For this review, take the finished solid that the model builds, in its own axes (mm). A direction names the side the tool comes from. Round coordinates to 2 decimals unless told otherwise and drop trailing zeros. Write each loop counter-clockwise with the first axis right and the second up, starting at its lowest first coordinate (ties: lowest second). Pieces come first, ordered by that corner, then holes. Notation, with made-up numbers: (39, 47.5) -> (50, 47.5) arc R19 ccw to (50, 60.5) -> close; hole circle Ø1 at (32.5, 40). An arc over 180 degrees is marked (long way). Answer in a Markdown table with one row per item.
from build123d import *

# Parameters (mm, degrees)
F1_DEPTH = 12.7
F3_DEPTH = 1.27
F4_DEPTH = 1.27
F5_W     = 15.24
F5_H     = 2.54
F6_DEPTH = 19.05


with BuildPart() as f1:
    # F0 (on Front) → F1 (new body, symmetric)
    with BuildSketch(Plane.XZ):
        Polygon((-22.86, 14.2980794165), (-31.115, 0), (0, 0), (0, 14.2980794165), align=None)
        Polygon((0, 14.2980794165), (0, 0), (31.115, 0), (22.86, 14.2980794165), align=None)
        Polygon((0, 0), (0, -14.2980794165), (39.37, -14.2980794165), (31.115, 0), align=None)
        Polygon((-31.115, 0), (-39.37, -14.2980794165), (0, -14.2980794165), (0, 0), align=None)
    extrude(amount=F1_DEPTH, both=True)

    # F2 (on face) → F3 (cut)
    with BuildSketch(Plane.XZ.offset(12.7)):
        with BuildLine():
            Line((0, -11.0009658396), (-0.00127, -10.9987661351))
            ThreePointArc((-0.00127, -10.9987661351), (-0.0021997045, -10.9996958396), (-0.00254, -11.0009658396))
            Line((-0.00254, -11.0009658396), (0, -11.0009658396))
        make_face()
        with BuildLine():
            ThreePointArc((-6.34873, -0.0046429161), (-6.35, -0.0049832116), (-6.35127, -0.0046429161))
            Line((-6.35127, -0.0046429161), (-12.7, -11.0009658396))
            Line((-12.7, -11.0009658396), (-0.00254, -11.0009658396))
            ThreePointArc((-0.00254, -11.0009658396), (-0.0021997045, -10.9996958396), (-0.00127, -10.9987661351))
            Line((-0.00127, -10.9987661351), (-6.34873, -0.0046429161))
        make_face()
        with BuildLine():
            Line((-6.34873, -0.0046429161), (-6.35, -0.0024432116))
            Line((-6.35, -0.0024432116), (-6.35127, -0.0046429161))
            ThreePointArc((-6.35127, -0.0046429161), (-6.35, -0.0049832116), (-6.34873, -0.0046429161))
        make_face()
    extrude(amount=-F3_DEPTH, mode=Mode.SUBTRACT)

    # F2 (on face) → F4 (cut)
    with BuildSketch(Plane.XZ.offset(12.7)):
        with BuildLine():
            Line((6.34873, -0.0002435071), (0, 10.9960794165))
            Line((0, 10.9960794165), (-6.34873, -0.0002435071))
            ThreePointArc((-6.34873, -0.0002435071), (-6.3478002955, -0.0011732116), (-6.34746, -0.0024432116))
            Line((-6.34746, -0.0024432116), (6.34746, -0.0024432116))
            ThreePointArc((6.34746, -0.0024432116), (6.3478002955, -0.0011732116), (6.34873, -0.0002435071))
        make_face()
        with BuildLine():
            ThreePointArc((-6.34873, -0.0046429161), (-6.35, -0.0049832116), (-6.35127, -0.0046429161))
            Line((-6.35127, -0.0046429161), (-12.7, -11.0009658396))
            Line((-12.7, -11.0009658396), (-0.00254, -11.0009658396))
            ThreePointArc((-0.00254, -11.0009658396), (-0.0021997045, -10.9996958396), (-0.00127, -10.9987661351))
            Line((-0.00127, -10.9987661351), (-6.34873, -0.0046429161))
        make_face()
        with BuildLine():
            Line((12.7, -11.0009658396), (6.35127, -0.0046429161))
            ThreePointArc((6.35127, -0.0046429161), (6.35, -0.0049832116), (6.34873, -0.0046429161))
            Line((6.34873, -0.0046429161), (0.00127, -10.9987661351))
            ThreePointArc((0.00127, -10.9987661351), (0.0021997045, -10.9996958396), (0.00254, -11.0009658396))
            Line((0.00254, -11.0009658396), (12.7, -11.0009658396))
        make_face()
        with BuildLine():
            Line((-6.34873, -0.0046429161), (-6.35, -0.0024432116))
            Line((-6.35, -0.0024432116), (-6.35127, -0.0046429161))
            ThreePointArc((-6.35127, -0.0046429161), (-6.35, -0.0049832116), (-6.34873, -0.0046429161))
        make_face()
        with BuildLine():
            Line((-6.34746, -0.0024432116), (-6.35, -0.0024432116))
            Line((-6.35, -0.0024432116), (-6.34873, -0.0046429161))
            ThreePointArc((-6.34873, -0.0046429161), (-6.3478002955, -0.0037132116), (-6.34746, -0.0024432116))
        make_face()
        with BuildLine():
            ThreePointArc((-6.34746, -0.0024432116), (-6.3478002955, -0.0011732116), (-6.34873, -0.0002435071))
            Line((-6.34873, -0.0002435071), (-6.35, -0.0024432116))
            Line((-6.35, -0.0024432116), (-6.34746, -0.0024432116))
        make_face()
        with BuildLine():
            Line((6.35, -0.0024432116), (6.34873, -0.0002435071))
            ThreePointArc((6.34873, -0.0002435071), (6.3478002955, -0.0011732116), (6.34746, -0.0024432116))
            Line((6.34746, -0.0024432116), (6.35, -0.0024432116))
        make_face()
        with BuildLine():
            Line((6.34873, -0.0046429161), (6.35, -0.0024432116))
            Line((6.35, -0.0024432116), (6.34746, -0.0024432116))
            ThreePointArc((6.34746, -0.0024432116), (6.3478002955, -0.0037132116), (6.34873, -0.0046429161))
        make_face()
        with BuildLine():
            Line((6.35127, -0.0046429161), (6.35, -0.0024432116))
            Line((6.35, -0.0024432116), (6.34873, -0.0046429161))
            ThreePointArc((6.34873, -0.0046429161), (6.35, -0.0049832116), (6.35127, -0.0046429161))
        make_face()
        with BuildLine():
            Line((0, -11.0009658396), (-0.00127, -10.9987661351))
            ThreePointArc((-0.00127, -10.9987661351), (-0.0021997045, -10.9996958396), (-0.00254, -11.0009658396))
            Line((-0.00254, -11.0009658396), (0, -11.0009658396))
        make_face()
        with BuildLine():
            ThreePointArc((0.00127, -10.9987661351), (0, -10.9984258396), (-0.00127, -10.9987661351))
            Line((-0.00127, -10.9987661351), (0, -11.0009658396))
            Line((0, -11.0009658396), (0.00127, -10.9987661351))
        make_face()
        with BuildLine():
            ThreePointArc((0.00254, -11.0009658396), (0.0021997045, -10.9996958396), (0.00127, -10.9987661351))
            Line((0.00127, -10.9987661351), (0, -11.0009658396))
            Line((0, -11.0009658396), (0.00254, -11.0009658396))
        make_face()
    extrude(amount=-F4_DEPTH, mode=Mode.SUBTRACT)

    # F5 (on face) → F6 (cut)
    with BuildSketch(Plane.XY.offset(14.2980794165)):
        Rectangle(F5_W, F5_H)
    extrude(amount=-F6_DEPTH, mode=Mode.SUBTRACT)


solid = f1.part
1) Consider section B-B on y = 0.5. State the section outline as (x, z) points.
Solved:
| item | result |
|---|---|
| outline | (-39.37, -14.3) -> (39.37, -14.3) -> (22.86, 14.3) -> (7.62, 14.3) -> (7.62, -4.75) -> (-7.62, -4.75) -> (-7.62, 14.3) -> (-22.86, 14.3) -> close |
2) Clearance check with flat-ended pins moving along their axes: pin 1 Ø1.5 at (y, z) = (-6, 0) entering from +X; pin 2 Ø1.3 at (x, y) = (-3, -0.5) entering from +Z; pin 3 Ø3 at (y, z) = (4, -5) entering from -X. State where each tip first meets the part, or that it passes through.
Solved:
| item | result |
|---|---|
| pin 1 | x = 31.55 |
| pin 2 | z = -4.75 |
| pin 3 | x = -34.87 |
3) For faces 4 (the flat face through (3.22, -12.07, -5.42)), 5 (the flat face through (-7.62, 0, 5)), 6 (the flat face through (8, -12.7, 0)), list the 3-axis set-ups (+Z, -Z, +X, -X, +Y, -Y) from which the entire face can be reached by the end or side of a thin tool; tool diameter is ignored.
Solved:
| item | result |
|---|---|
| face 4 | -Y |
| face 5 | +Z |
| face 6 | +Z, -Z, +X, -X, -Y |
4) Consider section C-C on x = -4.5. State the section outline as (y, z) points.
Solved:
| item | result |
|---|---|
| outline | (-12.7, -14.3) -> (12.7, -14.3) -> (12.7, 14.3) -> (1.27, 14.3) -> (1.27, -4.75) -> (-1.27, -4.75) -> (-1.27, 14.3) -> (-12.7, 14.3) -> (-12.7, 3.2) -> (-11.43, 3.2) -> (-11.43, 0) -> (-12.7, 0) -> (-12.7, -3.21) -> (-11.43, -3.21) -> (-11.43, -11) -> (-12.7, -11) -> close |
5) For line 1 (Y direction, x = -4, z = 8.5); line 2 (X direction, y = 11, z = 9.5); line 3 (Z direction, x = -32.5, y = 8.75), list the stretches that pass through material, from the lowest coordinate up. Write a range as [from, to].
Solved:
| item | result |
|---|---|
| line 1 | [-12.7, -1.27], [1.27, 12.7] |
| line 2 | [-25.63, 25.63] |
| line 3 | [-14.3, -2.4] |
6) Consider section D-D on z = -8.75. State the section outline as (x, y) points, then the cut area to 3 significant figures.
Solved:
| item | result |
|---|---|
| outline | (-36.17, -12.7) -> (-11.4, -12.7) -> (-11.4, -11.43) -> (-1.3, -11.43) -> (-1.3, -12.7) -> (1.3, -12.7) -> (1.3, -11.43) -> (11.4, -11.43) -> (11.4, -12.7) -> (36.17, -12.7) -> (36.17, 12.7) -> (-36.17, 12.7) -> close |
| area | 1,810 mm² |
7) Consider section A-A on z = 0.75. State the section outline as (x, y) points.
Solved:
| item | result |
|---|---|
| outline | (-30.68, -12.7) -> (-5.92, -12.7) -> (-5.92, -11.43) -> (5.92, -11.43) -> (5.92, -12.7) -> (30.68, -12.7) -> (30.68, 12.7) -> (-30.68, 12.7) -> close; hole (-7.62, -1.27) -> (7.62, -1.27) -> (7.62, 1.27) -> (-7.62, 1.27) -> close |
8) Mouldability with a two-part tool opening along Z and no side actions: class faces 1 (the flat face through (0, 0, -4.752)), 2 (the flat face through (0, 1.27, 5)), 3 (the flat face through (-3.13, -12.07, -5.58)) as pulls with the +Z half, pulls with the -Z half, needs draft (parallel to the pull), parting line crosses it, or undercut.
Solved:
| item | result |
|---|---|
| face 1 | pulls with the +Z half |
| face 2 | needs draft |
| face 3 | undercut |
